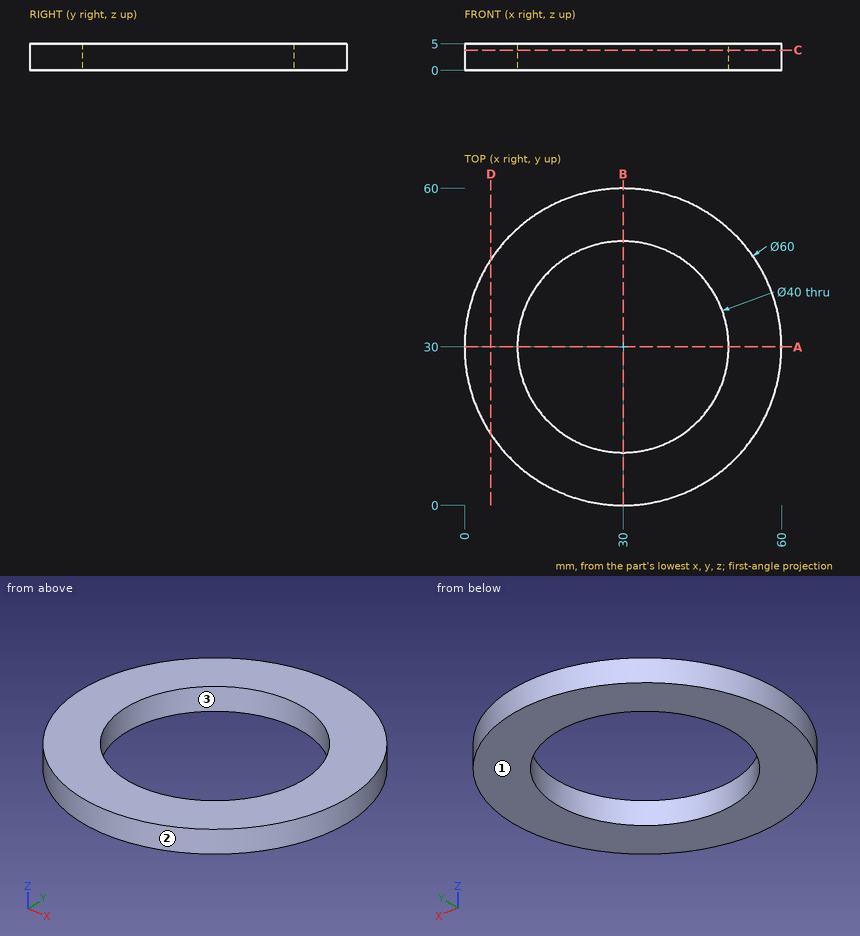
Source: three-view drawing plus pictorial views. Frame: mm from the lowest corner of the part. Give positions to 0.01 mm unless a question says otherwise; leave off trailing zeros. Loops run counter-clockwise (first coordinate to the right, second up) from the corner with the lowest first, then second, coordinate; pieces in that order, holes last. Notation, with made-up numbers: M 35.5,77 L 72.5,77 A32 cw 72.5,115 Z; hole C -20,-14 d11. An arc over 180 degrees is marked long. Use CSV: the item, a comma, the result in double quotes.
(1) Pull-direction query (Y, two-part tool) for the marked faces 1, 2 and 3; classes: pulls with the +Y half, pulls with the -Y half, needs draft (parallel to the pull), parting line crosses it, or undercut.
Outcome:
face 1,"needs draft"
face 2,"parting line crosses it"
face 3,"undercut"
(2) Section A-A, the plane y = 30. Return loops of the section in (x, z).
Outcome:
outline,"M 0,0 L 10,0 L 10,5 L 0,5 Z; M 50,0 L 60,0 L 60,5 L 50,5 Z"
(3) Section C-C, the plane z = 3.85. Return loops of the section in (x, y), plus the area to 3 significant figures.
Outcome:
outline,"C 30,30 d60; hole C 30,30 d40"
area,"1,570 mm²"
(4) Pin query (flat end, axial travel): P1, Ø1.5, axis at y = 24.5, z = 2, coming from the -X side; P2, Ø2, axis at x = 15.5, z = 1, coming from the -Y side; P3, Ø10, axis at x = 6.5, y = 37.5, coming from the -Z side. Return the tip coordinate at first contact, or that it passes through.
Outcome:
P1,"stops at x = 0.38"
P2,"stops at y = 3.21"
P3,"stops at z = 0"
(5) Section D-D, the plane x = 5. Return loops of the section in (y, z).
Outcome:
outline,"M 13.42,0 L 46.58,0 L 46.58,5 L 13.42,5 Z"
(6) Material intervals for L1, parallel to Y at x = 30, z = 1.5; L2, parallel to X at y = 24.5, z = 0.7; L3, parallel to Y at x = 20.5, z = 1.3, sorted ascending. Write a range as [from, to].
Outcome:
L1,"y = [0, 10], [50, 60]"
L2,"x = [0.51, 10.77], [49.23, 59.49]"
L3,"y = [1.54, 12.4], [47.6, 58.46]"
